Could you check a few things on this model? Use its own coordinates, in mm. A direction names the side the tool comes from. Give positions to 0.01 mm unless a question says otherwise; leave off trailing zeros. Write each loop counter-clockwise with the first axis right and the second up, starting at its lowest first coordinate (ties: lowest second). Pieces come first, ordered by that corner, then holes. Notation, with made-up numbers: (40.5, -37) - (46.5, -37) arc R21 cw to (46.5, -30) - close; hole circle Ø3 at (73.5, 35). An arc over 180 degrees is marked (long way). Answer in a Markdown table with one row per item.
from build123d import *

# Parameters (mm, degrees)
SKETCH_1_R           = 11
EXTRUDE_1_DEPTH      = 3.5
SKETCH_2_R           = 5
SKETCH_2_R_2         = 4
EXTRUDE_2_DEPTH      = 15
EXTRUDE_2_DEPTH_BACK = 5.5
SKETCH_3_R           = 4
SKETCH_3_R_2         = 1.75
CUT_EXTRUDE_1_DEPTH  = 6.5
CUT_EXTRUDE_2_DEPTH  = 10


with BuildPart() as part:
    # 草图1 → 凸台-拉伸1 (new body)
    with BuildSketch(Plane.XZ.offset(-1.5)):
        Circle(SKETCH_1_R)
    extrude(amount=-EXTRUDE_1_DEPTH)

    # 草图2 → 凸台-拉伸2 (add, two sides)
    with BuildSketch(Plane(origin=(0, 5, 0), x_dir=(1, 0, 0), z_dir=(0, 1, 0))) as extrude_2_sk:
        Circle(SKETCH_2_R)
        Circle(SKETCH_2_R_2, mode=Mode.SUBTRACT)
    extrude(amount=EXTRUDE_2_DEPTH)
    extrude(extrude_2_sk.sketch, amount=-EXTRUDE_2_DEPTH_BACK)

    # 草图3 → 切除-拉伸1 (cut, through all)
    with BuildSketch(Plane(origin=(0, 5, 0), x_dir=(1, 0, 0), z_dir=(0, 1, 0))):
        Circle(SKETCH_3_R)
        with Locations((-8, 0)):
            Circle(SKETCH_3_R_2)
        with Locations((0, 8)):
            Circle(SKETCH_3_R_2)
        with Locations((8, 0)):
            Circle(SKETCH_3_R_2)
        with Locations((0, -8)):
            Circle(SKETCH_3_R_2)
    extrude(amount=-CUT_EXTRUDE_1_DEPTH, mode=Mode.SUBTRACT)

    # 草图4 → 切除-拉伸2 (cut)
    with BuildSketch(Plane.XZ.offset(-1.5)):
        with BuildLine():
            Line((-6.25, -9.051933495), (-6.25, 9.051933495))
            ThreePointArc((-6.25, 9.051933495), (-11, 0), (-6.25, -9.051933495))
        make_face()
        with BuildLine():
            Line((6.25, 9.051933495), (6.25, -9.051933495))
            ThreePointArc((6.25, -9.051933495), (11, 0), (6.25, 9.051933495))
        make_face()
    extrude(amount=-CUT_EXTRUDE_2_DEPTH, mode=Mode.SUBTRACT)


solid = part.part
1) We'd pull the mould along Z, two halves only. Please class faces 1 (the face through (0, 3, 11)), 2 (the face through (-6.25, 3, 0)), 3 (the face through (1.617, 3.274, 8.67)): +Z half, -Z half, draft (parallel to the pull), parting line (faces both ways), or undercut.
Check values:
| item | result |
|---|---|
| face 1 | +Z half |
| face 2 | draft |
| face 3 | undercut |
2) Imagine slicing it at C-C (z = 0.5). List the corners of the cut face in (x, y) for me.
Check values:
| item | result |
|---|---|
| outline | (-6.25, 1.5) - (-4.97, 1.5) - (-4.97, -0.5) - (-3.97, -0.5) - (-3.97, 20) - (-4.97, 20) - (-4.97, 5) - (-6.25, 5) - close; (3.97, -0.5) - (4.97, -0.5) - (4.97, 1.5) - (6.25, 1.5) - (6.25, 5) - (4.97, 5) - (4.97, 20) - (3.97, 20) - close |
3) Will these pins go through, and if not, where does the flat tip stop? P1, Ø4, axis at x = 3.5, y = 10, coming from the -Z side; P2, Ø4, axis at x = 0, z = 8, coming from the -Y side; P3, Ø6, axis at x = 3.5, y = 2.5, coming from the +Z side.
Check values:
| item | result |
|---|---|
| P1 | stops at z = -4.77 |
| P2 | stops at y = 1.5 |
| P3 | stops at z = 10.99 |
4) If I drill on line 1 (Z direction, x = 0, y = 2.3); line 2 (X direction, y = 16, z = 0), over which ranges is the centre line in solid material (lowest first)?
Check values:
| item | result |
|---|---|
| line 1 | z = -11 to -9.75, -6.25 to -4, 4 to 6.25, 9.75 to 11 |
| line 2 | x = -5 to -4, 4 to 5 |
5) Imagine slicing it at B-B (y = 3.5). List the corners of the cut face in (x, z) for me.
Check values:
| item | result |
|---|---|
| outline | (-6.25, -9.05) arc R11 ccw to (6.25, -9.05) - (6.25, 9.05) arc R11 ccw to (-6.25, 9.05) - close; hole circle Ø8 at (0, 0); hole circle Ø3.5 at (0, -8); hole circle Ø3.5 at (0, 8) |
6) Imagine slicing it at A-A (x = 0). List the corners of the cut face in (y, z) for me, then the cut area to 3 significant figures.
Check values:
| item | result |
|---|---|
| outline | (-0.5, -5) - (1.5, -5) - (1.5, -6.25) - (5, -6.25) - (5, -5) - (20, -5) - (20, -4) - (-0.5, -4) - close; (-0.5, 4) - (20, 4) - (20, 5) - (5, 5) - (5, 6.25) - (1.5, 6.25) - (1.5, 5) - (-0.5, 5) - close; (1.5, -11) - (5, -11) - (5, -9.75) - (1.5, -9.75) - close; (1.5, 9.75) - (5, 9.75) - (5, 11) - (1.5, 11) - close |
| area | 58.5 mm2 |
7) On a 3-axis mill with a long thin cutter (end or side, diameter ignored), from which of +Z, -Z, +X, -X, +Y, -Y can I reach the whole of each face in a straight line? I mean faces 4 (the face through (6.25, 3, 0)), 5 (the face through (-1.08, 12.4, 4.88)), 6 (the face through (-1.5, 1.5, 5)). Say none if no direction works.
Check values:
| item | result |
|---|---|
| face 4 | +Z, -Z, +X, +Y, -Y |
| face 5 | +Y |
| face 6 | -Y |
8) Imagine slicing it at D-D (x = 3.5). List the corners of the cut face in (y, z) for me, then the cut area to 3 significant figures.
Check values:
| item | result |
|---|---|
| outline | (-0.5, -3.57) - (1.5, -3.57) - (1.5, -10.43) - (5, -10.43) - (5, -3.57) - (20, -3.57) - (20, -1.94) - (-0.5, -1.94) - close; (-0.5, 1.94) - (20, 1.94) - (20, 3.57) - (5, 3.57) - (5, 10.43) - (1.5, 10.43) - (1.5, 3.57) - (-0.5, 3.57) - close |
| area | 115 mm2 |
